Part model, mm, in its own coordinate system. A direction names the side the tool comes from. Coordinates: 2 decimals unless noted, no trailing zeros. Loops run counter-clockwise (first coordinate to the right, second up) from the corner with the lowest first, then second, coordinate; pieces in that order, holes last.
Autodesk Inventor part; units mm, degrees
ref_plane "YZ Plane" through (0, 0, 0) normal (1, 0, 0) x (0, 1, 0)
ref_plane "XZ Plane" through (0, 0, 0) normal (0, 1, 0) x (-1, 0, 0)
ref_plane "XY Plane" through (0, 0, 0) normal (0, 0, 1) x (1, 0, 0)
sketch "Sketch1" plane through (0, 0, 0) normal (0, 1, 0) x (-1, 0, 0)
  line L0 (161.2049, 265.4562) -> (-219.7951, 265.4562)
  line L1 (-219.7951, 265.4562) -> (-219.7951, -242.5438)
  line L2 (-219.7951, -242.5438) -> (161.2049, -242.5438)
  line L3 (161.2049, -242.5438) -> (161.2049, 265.4562)
  point P0 (0, 0)
  dimension "d0" = 508
  dimension "d1" = 381
extrude "Extrusion1" add sketch "Sketch1" along normal blind 25.4
sketch "Sketch2" plane through (0, 25.4, 0) normal (0, 1, 0) x (1, 0, 0)
  line L0 (-161.2049, -265.4562) -> (219.7951, -265.4562)
  line L1 (219.7951, -265.4562) -> (-161.2049, -265.4562)
  line L2 (-161.2049, 242.5438) -> (-161.2049, -265.4562)
  line L3 (-161.2049, -265.4562) -> (-161.2049, 242.5438)
  line L4 (219.7951, -265.4562) -> (219.7951, 242.5438)
  line L5 (-161.2049, 242.5438) -> (219.7951, 242.5438)
  line L6 (219.7951, 242.5438) -> (219.7951, -265.4562)
  line L7 (219.7951, -265.4562) -> (-161.2049, -265.4562)
  line L8 (219.7951, 242.5438) -> (-161.2049, 242.5438)
  line L9 (-161.2049, 242.5438) -> (219.7951, 242.5438)
  line L10 (-135.8049, -240.0562) -> (194.3951, -240.0562)
  line L11 (194.3951, -240.0562) -> (194.3951, 217.1438)
  line L12 (194.3951, 217.1438) -> (-135.8049, 217.1438)
  line L13 (-135.8049, 217.1438) -> (-135.8049, -240.0562)
  point P0 (0, 0)
  dimension "d4" = 25.4
extrude "Extrusion2" add sketch "Sketch2" along normal blind 228.6
sketch "Sketch4" plane through (0, 0, 0) normal (0, -1, 0) x (1, 0, 0)
  line L0 (-161.2049, 265.4562) -> (219.7951, 265.4562) construction
  line L1 (70.5701, 265.4562) -> (70.5701, -242.5438) construction
  line L2 (219.7951, -242.5438) -> (-161.2049, -242.5438) construction
  line L3 (219.7951, 265.4562) -> (219.7951, -242.5438) construction
  circle A0 centre (70.5701, 126.8865) radius 6.35
  circle A1 centre (70.5701, -103.9741) radius 6.35
  line L4 (-161.2049, -242.5438) -> (-161.2049, 265.4562) construction
  line L5 (-161.2049, 11.4562) -> (219.7951, 11.4562) construction
  point P0 (0, 0)
  dimension "d8" = 149.225
  dimension "d9" = 12.7
  dimension "d14" = 138.5697
  dimension "d15" = 138.5697
extrude "Extrusion3" cut sketch "Sketch4" against normal through all
equation "\"d14\" = d11"
equation "\"d11\" = d10"
properties part number "Battery Bucket"
Q1. Saw through at C-C (x = 136). List the corners of the cut face in (y, z).
Q2. Drop flat-ended pins along their axis: P1, Ø16.5, axis at x = 70.57, z = 126.89, coming from the +Y side; P2, Ø4, axis at x = -3, z = -50, coming from the -Y side. Give the stop position or say it passes through.
Q3. Saw through at A-A (z = -86.5). List the corners of the cut face in (x, y), plus the area to 3 significant figures.
Q4. Saw through at B-B (y = 195.5). List the corners of the cut face in (x, z), plus the area to 3 significant figures.
Q5. Probe line 1 (X direction, y = 217, z = -5); line 2 (Z direction, x = 179, y = 68); line 3 (Y direction, x = 16, z = 91). List the from-to ranges inside material, lowest first.
Q6. Mould opens along X. For faces 1 (the flat face through (194.395, 138, 15)), 2 (the flat face through (27, 125, 265.456)), 3 (the flat face through (219.795, 125, 15)) say: released by +X, released by -X, zero draft, split by the parting line, or undercut.
Q7. Tool access for faces 4 (the flat face through (32, 138, -217.144)), 5 (the flat face through (32, 125, -242.544)): list every direction of +Z, -Z, +X, -X, +Y, -Y with a clear straight run to the whole face (end or side of a thin tool).
Checked values:
1. outline: (0, -242.54) - (254, -242.54) - (254, -217.14) - (25.4, -217.14) - (25.4, 240.06) - (254, 240.06) - (254, 265.46) - (0, 265.46) - close
2. P1: stops at y = 25.4
2. P2: stops at y = 0
3. outline: (-161.2, 0) - (219.8, 0) - (219.8, 254) - (194.4, 254) - (194.4, 25.4) - (-135.8, 25.4) - (-135.8, 254) - (-161.2, 254) - close
3. area: 21,300 mm2
4. outline: (-161.2, -242.54) - (219.8, -242.54) - (219.8, 265.46) - (-161.2, 265.46) - close; hole (-135.8, -217.14) - (194.4, -217.14) - (194.4, 240.06) - (-135.8, 240.06) - close
4. area: 42,600 mm2
5. line 1: x = -161.2 to -135.8, 194.4 to 219.8
5. line 2: z = -242.54 to -217.14, 240.06 to 265.46
5. line 3: y = 0 to 25.4
6. face 1: undercut
6. face 2: zero draft
6. face 3: released by +X
7. face 4: +Y
7. face 5: -Z, +X, -X, +Y, -Y
